Input: part model. Units: mm. Frame: model coordinates. Face numbers are marked on the shaded views. Coordinates: 2 decimals unless noted, no trailing zeros. Order: outer loops, then holes, each group sorted by start corner. A loop starts at its lowest first (then second) coordinate and runs counter-clockwise, first axis right, second up. Notation, with made-up numbers: (-14, 31) -> (35, 31) arc R21 cw to (35, 36) -> close; hole circle Ø2 at (42, 7). An arc over 180 degrees is marked (long way). Write each question's results on one line, items separated by ' | '.
```python
from build123d import *

# Parameters (mm, degrees)
F0_R     = 12.7
F1_DEPTH = 101.6
F2_D     = 19.05
F3_D     = 19.05


with BuildPart() as f1:
    # F0 (on Front) → F1 (new body, symmetric)
    with BuildSketch(Plane.XZ):
        Circle(F0_R)
    extrude(amount=F1_DEPTH, both=True)

    # F2 (through all)
    with Locations(Plane(origin=(0, 0, 0), x_dir=(1, 0, 0), z_dir=(0, 1, 0))):
        with Locations((0, 0)):
            Hole(F2_D / 2)

    # F3 (through all)
    with Locations(Plane.XZ):
        with Locations((0, 0)):
            Hole(F3_D / 2)


solid = f1.part
```
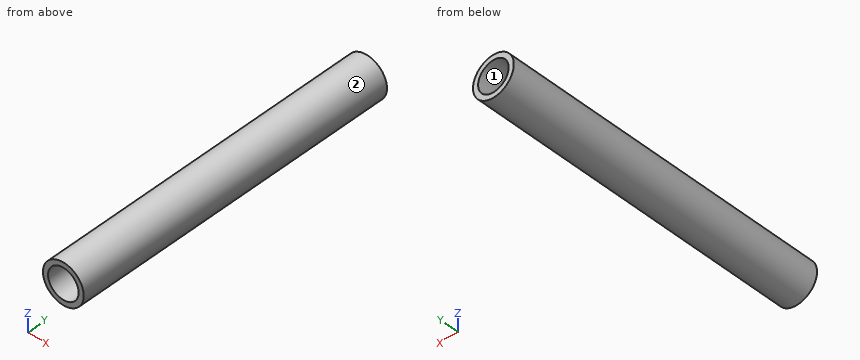
(1) Line query: line 1 along Z through (x, y) = (0, -16.5) (3 decimals); line 2 along X through (y, z) = (41, -0.75); line 3 along Z through (x, y) = (-8.75, -1). Output: solid intervals per line, ascending. Write a range as from..to.
Return value:
line 1: -12.7..-9.525, 9.525..12.7 | line 2: -12.68..-9.5, 9.5..12.68 | line 3: -9.2..-3.76, 3.76..9.2
(2) Cut plane C-C, the plane y = 0. Return loops of the section in (x, z) (3 decimals), plus the area to 3 significant figures.
Return value:
outline: circle Ø25.4 at (0, 0); hole circle Ø19.05 at (0, 0) | area: 222 mm2
(3) Mould query, pull axis X, two halves, no side actions, for the marked faces 1 and 2. Classes: +X half, -X half, draft (parallel to the pull), parting line (faces both ways), or undercut.
Return value:
face 1: undercut | face 2: parting line
(4) Cut plane A-A, the plane z = 0. Return loops of the section in (x, y) (3 decimals).
Return value:
outline: (-12.7, -101.6) -> (-9.525, -101.6) -> (-9.525, 101.6) -> (-12.7, 101.6) -> close; (9.525, -101.6) -> (12.7, -101.6) -> (12.7, 101.6) -> (9.525, 101.6) -> close
(5) Cut plane B-B, the plane x = 0. Return loops of the section in (y, z) (3 decimals).
Return value:
outline: (-101.6, -12.7) -> (101.6, -12.7) -> (101.6, -9.525) -> (-101.6, -9.525) -> close; (-101.6, 9.525) -> (101.6, 9.525) -> (101.6, 12.7) -> (-101.6, 12.7) -> close
(6) Pin query (flat end, axial travel): P1, Ø2, axis at x = -1, y = 24.5, coming from the +Z side; P2, Ø6, axis at y = 20.5, z = -6, coming from the +X side; P3, Ø3, axis at x = -8, y = 45.5, coming from the -Z side; P4, Ø4, axis at x = 4, y = -38.5, coming from the -Z side. Return the tip coordinate at first contact, or that it passes through.
Return value:
P1: z = 12.7 | P2: x = 12.34 | P3: z = -10.91 | P4: z = -12.54
